Geometry check sheet. Reference: the model listing, model coordinates, mm. Coordinates: 2 decimals unless noted, no trailing zeros. Write each loop counter-clockwise with the first axis right and the second up, starting at its lowest first coordinate (ties: lowest second). Pieces come first, ordered by that corner, then holes. Notation, with made-up numbers: (-36.5, 28) -> (16.5, 28) arc R24 cw to (16.5, 64) -> close; hole circle Ø5 at (27.5, -19.5). An arc over 180 degrees is marked (long way). Put each result on its own line as item: value. Start each with the question number.
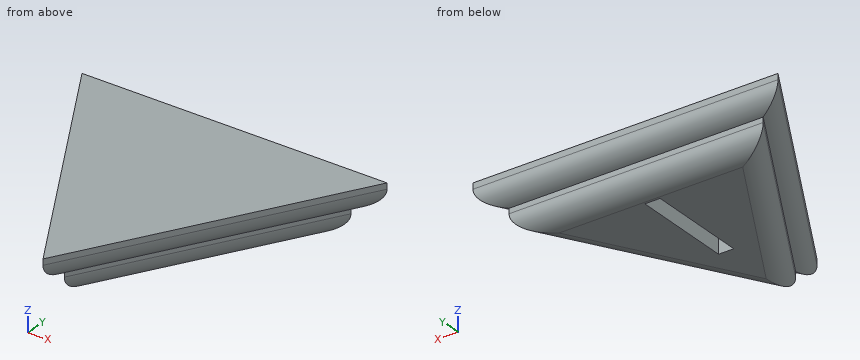
from build123d import *

# Parameters (mm, degrees)
F0_W         = 3
F0_H         = 20
F1_DEPTH     = 10
F2_DEPTH     = 5
F3_T1_DEPTH  = 70
F3_T3_DEPTH  = 79.20981353
F3_T5_DEPTH  = 70
F3_T7_DEPTH  = 70
F3_T9_DEPTH  = 79.20981353
F3_T11_DEPTH = 79.20981353


# Not quite as in the source:
# - a fillet or chamfer that OpenCascade refuses, or shapes differently, is made with other operations: its cross-section is extruded or revolved along the edge and cut away or added


with BuildPart() as f1:
    # F0 (on Top) → F1 (new body)
    with BuildSketch(Plane.XY):
        Polygon((25, 14.4337567297), (-25, 14.4337567297), (0, -28.8675134595), align=None)
        Rectangle(F0_W, F0_H, mode=Mode.SUBTRACT)
    extrude(amount=-F1_DEPTH)

    # F0 (on Top) → F2 (join)
    with BuildSketch(Plane.XY):
        Polygon((30, 17.3205080757), (-30, 17.3205080757), (0, -34.6410161514), align=None)
        Polygon((0, -28.8675134595), (-25, 14.4337567297), (25, 14.4337567297), align=None, mode=Mode.SUBTRACT)
        Rectangle(F0_W, F0_H)
    extrude(amount=-F2_DEPTH)

    # F3: fillet of radius 4 on 6 edges, made by hand

    # F3_s2 → F3_t1 (cut)
    with BuildSketch(Plane.YZ.offset(-35)):
        with BuildLine():
            ThreePointArc((14.4337567297, -6), (13.2621838545, -8.8284271247), (10.4337567297, -10))
            Line((10.4337567297, -10), (14.4337567297, -10))
            Line((14.4337567297, -10), (14.4337567297, -6))
        make_face()
    extrude(amount=F3_T1_DEPTH, mode=Mode.SUBTRACT)

    # F3_s4 → F3_t3 (cut)
    with BuildSketch(Plane.YZ.offset(-39.604906765)):
        with BuildLine():
            ThreePointArc((14.4337567297, -5), (16.5183975841, -3.5608487081), (17.3205080757, -1.158037294))
            Line((17.3205080757, -1.158037294), (17.3205080757, -5))
            Line((17.3205080757, -5), (14.4337567297, -5))
        make_face()
    extrude(amount=F3_T3_DEPTH, mode=Mode.SUBTRACT)

    # F3_s6 → F3_t5 (cut)
    with BuildSketch(Plane(origin=(-17.5, -30.3108891325, 0), x_dir=(0, 0, 1), z_dir=(0.5, 0.8660254038, 0))):
        with BuildLine():
            ThreePointArc((-10, 10.4337567297), (-8.8284271247, 13.2621838545), (-6, 14.4337567297))
            Line((-6, 14.4337567297), (-10, 14.4337567297))
            Line((-10, 14.4337567297), (-10, 10.4337567297))
        make_face()
    extrude(amount=F3_T5_DEPTH, mode=Mode.SUBTRACT)

    # F3_s8 → F3_t7 (cut)
    with BuildSketch(Plane(origin=(-17.5, 30.3108891325, 0), x_dir=(0, 0, 1), z_dir=(0.5, -0.8660254038, 0))):
        with BuildLine():
            ThreePointArc((-6, 14.4337567297), (-8.8284271247, 13.2621838545), (-10, 10.4337567297))
            Line((-10, 10.4337567297), (-10, 14.4337567297))
            Line((-10, 14.4337567297), (-6, 14.4337567297))
        make_face()
    extrude(amount=F3_T7_DEPTH, mode=Mode.SUBTRACT)

    # F3_s10 → F3_t9 (cut)
    with BuildSketch(Plane(origin=(-19.8024533825, -34.298855373, 0), x_dir=(0, 0, 1), z_dir=(0.5, 0.8660254038, 0))):
        with BuildLine():
            ThreePointArc((-5, 14.4337567297), (-3.5608487081, 16.5183975841), (-1.158037294, 17.3205080757))
            Line((-1.158037294, 17.3205080757), (-5, 17.3205080757))
            Line((-5, 17.3205080757), (-5, 14.4337567297))
        make_face()
    extrude(amount=F3_T9_DEPTH, mode=Mode.SUBTRACT)

    # F3_s12 → F3_t11 (cut)
    with BuildSketch(Plane(origin=(-19.8024533825, 34.298855373, 0), x_dir=(0, 0, 1), z_dir=(0.5, -0.8660254038, 0))):
        with BuildLine():
            ThreePointArc((-5, 14.4337567297), (-3.5608487081, 16.5183975841), (-1.158037294, 17.3205080757))
            Line((-1.158037294, 17.3205080757), (-5, 17.3205080757))
            Line((-5, 17.3205080757), (-5, 14.4337567297))
        make_face()
    extrude(amount=F3_T11_DEPTH, mode=Mode.SUBTRACT)


solid = f1.part
Item 1: Section check A-A, the plane z = -7.5. Enter the section's corners in (x, y).
Item 2: Scan lines: line 1 along X through (y, z) = (-3.5, -6.25); line 2 along X through (y, z) = (6, -9.5); line 3 along Y through (x, z) = (-21, -7.75). Record each from-to range of solid material in increasing order. Write a range as [from, to].
Item 3: Go/stop test with flat-tipped pins: P1, Ø0.9, axis at x = -0.5, y = 2.5, coming from the -Z side; P2, Ø1.5, axis at y = -2, z = -7.5, coming from the +X side; P3, Ø3, axis at x = 22, z = -4, coming from the +Y side. Record where each tip stops, or that it passes through.
Item 4: Section check B-B, the plane z = -2. Enter the section's corners in (x, y), and give its area (3 significant figures).
From the geometry:
1. outline: (-24.49, 14.14) -> (0, -28.28) -> (24.49, 14.14) -> close; hole (-1.5, -10) -> (1.5, -10) -> (1.5, 10) -> (-1.5, 10) -> close
2. line 1: [-14.64, -1.5], [1.5, 14.64]
2. line 2: [-17.75, -1.5], [1.5, 17.75]
2. line 3: [8.31, 14.03]
3. P1: z = -5
3. P2: x = 15.7
3. P3: y = 17.09
4. outline: (-29.84, 17.23) -> (0, -34.46) -> (29.84, 17.23) -> close
4. area: 1,540 mm²
